```python
from build123d import *

# Parameters (mm, degrees)
SKETCH1_R          = 34.925
SKETCH1_R_2        = 8
BASE_EXTRUDE_DEPTH = 12.7
SKETCH6_R          = 3.3655
CUT_EXTRUDE1_DEPTH = 51.998051433
CIRPATTERN2_COUNT  = 6
SKETCH11_R         = 23.07124837
CUT_EXTRUDE3_DEPTH = 2
SKETCH12_R         = 11.5
CUT_EXTRUDE4_DEPTH = 2
SKETCH14_R         = 17.4625
CUT_EXTRUDE5_DEPTH = 51.998051433


with BuildPart() as part:
    # Sketch1 → Base-Extrude (new body)
    with BuildSketch(Plane.XY):
        Circle(SKETCH1_R)
        Circle(SKETCH1_R_2, mode=Mode.SUBTRACT)
    extrude(amount=BASE_EXTRUDE_DEPTH)

    # Sketch6 → Cut-Extrude1 (cut, through all)
    with BuildSketch(Plane(origin=(0, 0, 0), x_dir=(-1, 0, 0), z_dir=(0, 0, -1))):
        with Locations((0, 29.3624)):
            Circle(SKETCH6_R)
    cut_extrude1 = extrude(amount=-CUT_EXTRUDE1_DEPTH, mode=Mode.SUBTRACT)

    # CirPattern2: Cut-Extrude1 ×6 about axis
    cirpattern2_axis = Axis((0, 0, 0), (0, 0, 1))
    for i in range(1, CIRPATTERN2_COUNT):
        add(cut_extrude1.rotate(cirpattern2_axis, i * 360 / CIRPATTERN2_COUNT), mode=Mode.SUBTRACT)

    # Sketch11 → Cut-Extrude3 (cut)
    with BuildSketch(Plane(origin=(0, 0, 0), x_dir=(-1, 0, 0), z_dir=(0, 0, -1))):
        Circle(SKETCH11_R)
    extrude(amount=-CUT_EXTRUDE3_DEPTH, mode=Mode.SUBTRACT)

    # Sketch12 → Cut-Extrude4 (cut)
    with BuildSketch(Plane.XY.offset(12.7)):
        Circle(SKETCH12_R)
    extrude(amount=-CUT_EXTRUDE4_DEPTH, mode=Mode.SUBTRACT)

    # Sketch14 → Cut-Extrude5 (cut, through all)
    with BuildSketch(Plane.XY.offset(12.7)):
        Circle(SKETCH14_R)
    extrude(amount=-CUT_EXTRUDE5_DEPTH, mode=Mode.SUBTRACT)


solid = part.part
```
The listing builds one solid part. Answer for the finished solid, in the listing's coordinates (mm). A direction names the side the tool comes from. Give positions to 0.01 mm unless a question says otherwise; leave off trailing zeros. Order: outer loops, then holes, each group sorted by start corner. A loop starts at its lowest first (then second) coordinate and runs counter-clockwise, first axis right, second up. Notation, with made-up numbers: M 45,37 L 80,37 A18 ccw 80,67 Z; hole C 17,38 d3. An arc over 180 degrees is marked long. Put each result on its own line as item: value. Start each with the question number.
Item 1: The part is cut by section C-C, the plane z = 6.25. State how many separate pieces and enclosed holes the cut face has, and give its area (3 significant figures).
Item 2: The part is cut by section B-B, the plane y = 0. Determine the outline of the cut face in (x, z) (1 decimal).
Item 3: Flat-ended cylindrical pins translate along their axes: P1, Ø5, axis at y = 24.5, z = 1.5, coming from the +X side; P2, Ø2, axis at x = 17.5, z = 2.5, coming from the -Y side; P3, Ø2, axis at x = -8, z = 10.5, coming from the -Y side. Find the tip coordinate at first contact, or state that the pin passes through.
Item 4: For a pull along X with two mould halves and no side action, classify faces 3 (the face through (-0.73, -26.077, 6.261)), 4 (the face through (-27.715, -21.251, 6.261)), 5 (the face through (-8, 16, 12.7)), 6 (the face through (-8.4, 15.5, 2)) as +X half, -X half, draft (parallel to the pull), parting line (faces both ways), or undercut.
Item 5: The part is cut by section D-D, the plane y = -14.5. Determine the outline of the cut face in (x, z).
Item 6: Which of the six approach directions +Z, -Z, +X, -X, +Y, -Y give full straight-line access (tool end or side, diameter ignored) to faces 1 (the face through (-13.858, -10.626, 7.425)), 2 (the face through (-12.403, 19.454, 0.986))?
Item 7: The part is cut by section A-A, the plane x = 0. Determine the outline of the cut face in (y, z) (1 decimal).
Item 8: Find the intervals of material crossed by line 1 along Y through (x, z) = (0, 10) (1 decimal); line 2 along X through (y, z) = (-13, 11.75); line 3 along X through (y, z) = (14.5, 7.5), in increasing order.
Answer key:
1. separate pieces: 1
1. enclosed holes: 7
1. area: 2,660 mm²
2. outline: M -34.9,0 L -23.1,0 L -23.1,2 L -17.5,2 L -17.5,12.7 L -34.9,12.7 Z; M 17.5,2 L 23.1,2 L 23.1,0 L 34.9,0 L 34.9,12.7 L 17.5,12.7 Z
3. P1: stops at x = 27.12
3. P2: stops at y = -30.78
3. P3: stops at y = -34.22
4. face 3: undercut
4. face 4: parting line
4. face 5: draft
4. face 6: undercut
5. outline: M -31.77,0 L -28.79,0 L -28.79,12.7 L -31.77,12.7 Z; M -22.07,0 L -17.95,0 L -17.95,2 L -9.73,2 L -9.73,12.7 L -22.07,12.7 Z; M 9.73,2 L 17.95,2 L 17.95,0 L 22.07,0 L 22.07,12.7 L 9.73,12.7 Z; M 28.79,0 L 31.77,0 L 31.77,12.7 L 28.79,12.7 Z
6. face 1: +Z, -Z
6. face 2: -Z
7. outline: M -34.9,0 L -32.7,0 L -32.7,12.7 L -34.9,12.7 Z; M -26,0 L -23.1,0 L -23.1,2 L -17.5,2 L -17.5,12.7 L -26,12.7 Z; M 17.5,2 L 23.1,2 L 23.1,0 L 26,0 L 26,12.7 L 17.5,12.7 Z; M 32.7,0 L 34.9,0 L 34.9,12.7 L 32.7,12.7 Z
8. line 1: y = -34.9 to -32.7, -26 to -17.5, 17.5 to 26, 32.7 to 34.9
8. line 2: x = -32.42 to -28.34, -22.51 to -11.66, 11.66 to 22.51, 28.34 to 32.42
8. line 3: x = -31.77 to -28.79, -22.07 to -9.73, 9.73 to 22.07, 28.79 to 31.77
